Part print with two shaded views. Sizes in mm from the minimum x, y, z corner. A direction names the side the tool comes from. Give positions to 0.01 mm unless a question says otherwise; leave off trailing zeros. Order: outer loops, then holes, each group sorted by start corner. A loop starts at its lowest first (then second) coordinate and runs counter-clockwise, first axis right, second up. Notation, with made-up numbers: (60, 13) -> (81, 13) arc R18 cw to (81, 37) -> close; hole circle Ø10 at (89.25, -24). An arc over 180 degrees is marked (long way). Write item = value, one per line. Start each with the question number.
Item 1: Flat gauge pins, fed straight in: P1, Ø8, axis at x = 33.5, y = 14.5, coming from the -Z side; P2, Ø5, axis at x = 17, y = 15, coming from the +Z side; P3, Ø1.9, axis at x = 18.5, y = 15, coming from the -Z side. Where does each tip first touch, or does it go through?
Item 2: Drill centre lines: line 1 along X through (y, z) = (22.25, 5.25); line 2 along Y through (x, z) = (3.5, 23.5); line 3 along Z through (x, y) = (16.5, 15.75). Where is each one in solid material? Low to high.
Item 3: Band-saw the part on A-A on z = 5. Write the cut outline in (x, y).
Item 4: Band-saw the part on B-B on x = 26. Write the cut outline in (y, z).
Item 5: Tool access for the marked faces 5, 6 and 7: list every direction of +Z, -Z, +X, -X, +Y, -Y with a clear straight run to the whole face (end or side of a thin tool).
Item 6: Pull direction X, two halves, no side cores. Call the marked faces 1, 2, 3 and 4: +X half, -X half, draft (parallel to the pull), parting line (faces both ways), or undercut.
Item 7: Band-saw the part on D-D on y = 14.75. Write the cut outline in (x, z).
Item 8: Band-saw the part on C-C on z = 20.25. Write the cut outline in (x, y), plus the area to 3 significant figures.
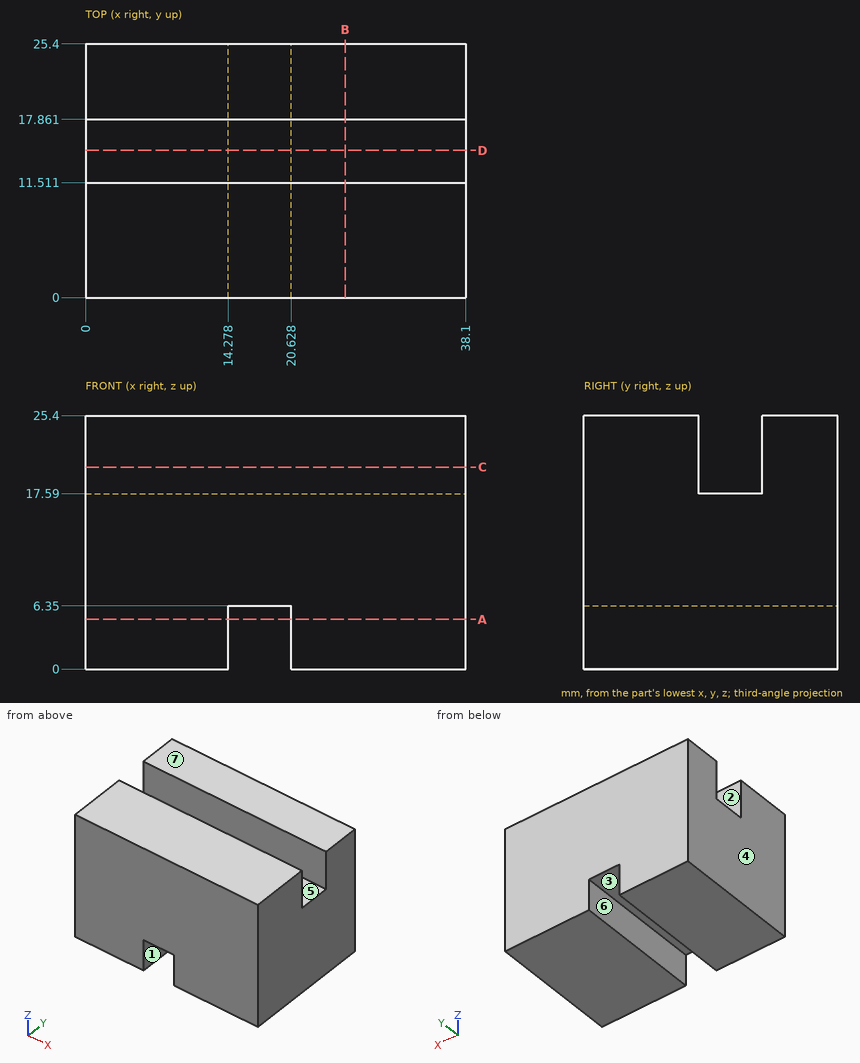
Values found:
q1.P1 = 0
q1.P2 = 17.59
q1.P3 = 6.35
q2.line_1 = 0 to 14.28, 20.63 to 38.1
q2.line_2 = 0 to 11.51, 17.86 to 25.4
q2.line_3 = 6.35 to 17.59
q3.outline = (0, 0) -> (14.28, 0) -> (14.28, 25.4) -> (0, 25.4) -> close; (20.63, 0) -> (38.1, 0) -> (38.1, 25.4) -> (20.63, 25.4) -> close
q4.outline = (0, 0) -> (25.4, 0) -> (25.4, 25.4) -> (17.86, 25.4) -> (17.86, 17.59) -> (11.51, 17.59) -> (11.51, 25.4) -> (0, 25.4) -> close
q5.face_5 = +Z, +X, -X
q5.face_6 = -Z, +Y, -Y
q5.face_7 = +Z, +X, -X, +Y, -Y
q6.face_1 = undercut
q6.face_2 = draft
q6.face_3 = undercut
q6.face_4 = -X half
q7.outline = (0, 0) -> (14.28, 0) -> (14.28, 6.35) -> (20.63, 6.35) -> (20.63, 0) -> (38.1, 0) -> (38.1, 17.59) -> (0, 17.59) -> close
q8.outline = (0, 0) -> (38.1, 0) -> (38.1, 11.51) -> (0, 11.51) -> close; (0, 17.86) -> (38.1, 17.86) -> (38.1, 25.4) -> (0, 25.4) -> close
q8.area = 726 mm^2
